Work out the finished part from the listing and answer in its coordinate system (mm). Give positions to 0.01 mm unless a question says otherwise; leave off trailing zeros. Write each loop counter-clockwise with the first axis right and the second up, starting at its lowest first coordinate (ties: lowest second). Pieces come first, ordered by that corner, then holes.
1) Determine the mould class of faces 1 (the face through (-134.76, 1.97, -18.33)), 2 (the face through (-8.294, 1.972, 8.848)), 3 (the face through (-71, 0, -12)) for opening direction X: pulls with the +X half, pulls with the -X half, needs draft (parallel to the pull), parting line crosses it, or undercut.
2) Given pin 1 Ø11 at (x, z) = (-130, -14.678) entering from +Y; pin 2 Ø1.5 at (x, y) = (-84.5, 2) entering from -Z, each flat-ended and moving along its own axis, determine where each tip first touches the part or whether it passes through.
3) Find section C-C (y = 1.2). Determine the outline of the cut face in (x, z).
4) Find section B-B (z = -18.5). Determine the outline of the cut face in (x, y).
5) Straight lines are drawn through the part: probe 1 along Z at (x, y) = (-130, 2.1); probe 2 along Z at (x, y) = (-15.5, 2); probe 3 along Z at (x, y) = (-59, 0.65). For each, find the intervals that lie inside material, in ascending order.
6) Find section A-A (x = -20). Determine the outline of the cut face in (y, z).
7) Find section D-D (z = -29). Determine the outline of the cut face in (x, y), plus the area to 3 significant figures.
Autodesk Inventor part; units mm, degrees
ref_plane "YZ Plane" through (0, 0, 0) normal (1, 0, 0) x (0, 1, 0)
ref_plane "XZ Plane" through (0, 0, 0) normal (0, 1, 0) x (-1, 0, 0)
ref_plane "XY Plane" through (0, 0, 0) normal (0, 0, 1) x (1, 0, 0)
sketch "スケッチ1" plane through (0, 0, 0) normal (0, 1, 0) x (-1, 0, 0)
  arc A0 (209.8798, -23.6971) -> (38.3003, 12.1023) centre (-36.3979, -774.9853) ccw
  arc A1 (99.4686, -35.9265) -> (209.8798, -23.6971) centre (88.5018, 567.6156) ccw
  arc A2 (73.7238, -35.6322) -> (99.4686, -35.9265) centre (91.566, 398.982) ccw
  arc A3 (26.4399, -27.2272) -> (73.7238, -35.6322) centre (81.048, 142.776) ccw
  arc A4 (-0.8557, -13.8205) -> (26.4399, -27.2272) centre (58.458, 72.45) ccw
  arc A5 (-8.6045, -6.2961) -> (-0.8557, -13.8205) centre (17.4, 12.732) ccw
  arc A6 (-1.8835, 10.4943) -> (-8.6045, -6.2961) centre (0, 0) ccw
  arc A7 (18.284, 12.3227) -> (-1.8835, 10.4943) centre (18.66, -103.968) ccw
  arc A8 (38.3003, 12.1023) -> (18.284, 12.3227) centre (20.556, -690.396) ccw
extrude "押し出し1" add sketch "スケッチ1" along normal blind 4
sketch "スケッチ2" plane through (0, 0, 0) normal (0, -1, 0) x (1, 0, 0)
  circle A0 centre (-20, -2.2582) radius 6
  circle A1 centre (-130, -14.678) radius 6
  line L0 (0, 0) -> (-209.8798, -23.6971)
  dimension "d3" = 12
  dimension "d4" = 12
  dimension "d5" = 20
  dimension "d6" = 130
extrude "押し出し2" cut sketch "スケッチ2" against normal through all
thicken "厚み1" operation cut thickness 3 both sides no extend neighbours no toward (0.2114907, 0, -0.97738) faces at (-130.8117, 2.6667, -2.245) (-36.0766, 2.6667, 12.1549) (-0.3377, 1.3333, 10.8708) (9.052, 1.3333, -5.6337) (1.8363, 1.3333, -13.1189) (-10.787, 2.6667, -20.7604) (-68.3801, 1.3333, -35.3326) (-85.1636, 2.6667, -35.9512) (-200.7848, 1.3333, -25.4914)
equation "\"d4\" = d3"
properties part number "plate" material "木材 (オーク)"
Results:
1. face 1: undercut
1. face 2: pulls with the +X half
1. face 3: needs draft
2. pin 1: passes through
2. pin 2: stops at z = -32.95
3. outline: (-197.82, -22.99) arc R600.64 ccw to (-99.41, -32.93) arc R431.99 ccw to (-73.85, -32.63) arc R175.56 ccw to (-27.36, -24.37) arc R101.69 ccw to (-0.84, -11.35) arc R29.22 ccw to (6.18, -4.52) arc R7.66 ccw to (1.35, 7.54) arc R113.28 ccw to (-18.29, 9.32) arc R699.76 ccw to (-38.02, 9.11) arc R787.63 ccw to start; hole circle Ø12 at (-130, -14.68); hole circle Ø12 at (-20, -2.26)
4. outline: (-182.88, 0) - (-134.63, 0) - (-134.63, 4) - (-182.88, 4) - close; (-125.37, 0) - (-12.96, 0) - (-12.96, 4) - (-125.37, 4) - close
5. probe 1: z = -31.59 to -20.68, -8.68 to -5.14
5. probe 2: z = -19.72 to -6.23, 1.71 to 9.28
5. probe 3: z = -31.39 to 6.84
6. outline: (0, -21.69) - (4, -21.69) - (4, -8.26) - (0, -8.26) - close; (0, 3.74) - (4, 3.74) - (4, 9.33) - (0, 9.33) - close
7. outline: (-157.93, 0) - (-44.8, 0) - (-44.8, 4) - (-157.93, 4) - close
7. area: 453 mm2
